The listing builds one solid part. Answer for the finished solid, in the listing's coordinates (mm). A direction names the side the tool comes from. Round coordinates to 2 decimals unless told otherwise and drop trailing zeros. Order: outer loops, then holes, each group sorted by start corner. A loop starts at its lowest first (then second) coordinate and runs counter-clockwise, first axis right, second up. Notation, with made-up numbers: (-17, 18.5) -> (19, 18.5) arc R30 cw to (19, 47.5) -> close; hole circle Ø4 at (47, 45.25). An arc over 180 degrees is marked (long way). Return JSON: item names as keys, results as strings. Group by question number.
(1) The part is cut by section D-D (z = 20.01). Determine the outline of the cut face in (x, y).
(2) Which of the six approach directions +Z, -Z, +X, -X, +Y, -Y give full straight-line access (tool end or side, diameter ignored) to faces 1 (the face through (0, 17, 17)), 2 (the face through (0, 3, -20)), 3 (the face through (0, 1, 17)), 4 (the face through (0.1, 5.9, 7.5)), 5 (the face through (0, 4.5, -20))?
(3) Each of these flat-tipped pins is pushed along its axis until it touches: pin 1 (2.5 mm diameter, centred on x = 3, z = 19, fed in from +Y); pin 2 (2.5 mm diameter, centred on x = -2, y = 1.5, fed in from -Z); pin 3 (1.8 mm diameter, centred on x = -4.55, z = 20.01, fed in from -Y); pin 4 (1 mm diameter, centred on x = -0.5, y = 27, fed in from +Z). Where does it stop, or does it pass through?
(4) The part is cut by section B-B (z = 10). Determine the outline of the cut face in (x, y), plus the area to 3 significant figures.
(5) The part is cut by section C-C (x = 0). Determine the outline of the cut face in (y, z).
(6) Consider line 1 (X direction, y = 3.7, z = 20.01); line 2 (Z direction, x = -0.75, y = 14.5); line 3 (X direction, y = 4.5, z = 10). Determine where each line is inside the solid, lowest interval first. Write a range as [from, to].
(7) Determine the mould class of faces 6 (the face through (6.724, 3.74, 19.527)), 7 (the face through (0, 4, 22)), 8 (the face through (5.56, 3.74, -21.12)) for opening direction X: +X half, -X half, draft (parallel to the pull), parting line (faces both ways), or undercut.
(8) The part is cut by section A-A (x = 4.55). Determine the outline of the cut face in (y, z).
from build123d import *

# Parameters (mm, degrees)
SKETCH1_W           = 14
SKETCH1_H           = 34
SKETCH1_R           = 2.5
BOSS_EXTRUDE1_DEPTH = 30
SKETCH1_3_R         = 2.5
CUT_EXTRUDE1_DEPTH  = 12
BOSS_EXTRUDE2_START = -3
SKETCH4_R           = 1.5
BOSS_EXTRUDE2_DEPTH = 1.5


with BuildPart() as part:
    # Sketch1 → Boss-Extrude1 (new body)
    with BuildSketch(Plane(origin=(0, 0, 0), x_dir=(1, 0, 0), z_dir=(0, 1, 0))):
        Rectangle(SKETCH1_W, SKETCH1_H)
        with Locations((0, -10)):
            Circle(SKETCH1_R, mode=Mode.SUBTRACT)
        with Locations((0, -10)):
            Circle(SKETCH1_R)
    extrude(amount=BOSS_EXTRUDE1_DEPTH)

    # Sketch1_3 → Cut-Extrude1 (cut)
    with BuildSketch(Plane(origin=(0, 0, 0), x_dir=(1, 0, 0), z_dir=(0, 1, 0))):
        with Locations(Location((0, -10, 0), (0, 0, 270))):
            Circle(SKETCH1_3_R)
    extrude(amount=CUT_EXTRUDE1_DEPTH, mode=Mode.SUBTRACT)

    # Sketch4 → Boss-Extrude2 (add)
    with BuildSketch(Plane.XZ.offset(BOSS_EXTRUDE2_START)):
        with BuildLine():
            Line((0, 22), (-5.877806956, 22))
            ThreePointArc((-5.877806956, 22), (-6.716005023, 19.562192285), (-7, 17))
            Line((-7, 17), (0, 17))
            Line((0, 17), (0, 22))
        make_face()
        with Locations(Location((-4.55, 20.01, 0), (0, 0, 270))):
            Circle(SKETCH4_R, mode=Mode.SUBTRACT)
        with BuildLine():
            Line((5.877806956, 22), (0, 22))
            Line((0, 22), (0, 17))
            Line((0, 17), (7, 17))
            ThreePointArc((7, 17), (6.716005023, 19.562192285), (5.877806956, 22))
        make_face()
        with Locations(Location((4.55, 20.01, 0), (0, 0, 270))):
            Circle(SKETCH4_R, mode=Mode.SUBTRACT)
    boss_extrude2 = extrude(amount=-BOSS_EXTRUDE2_DEPTH)

    # Mirror1: Boss-Extrude2 across plane
    add(boss_extrude2.mirror(Plane.XY))


solid = part.part
Answer below:
{
 "1": {"outline": "(-6.61, 3) -> (-6.05, 3) -> (-6.05, 4.5) -> (-6.61, 4.5) -> close; (-3.05, 3) -> (3.05, 3) -> (3.05, 4.5) -> (-3.05, 4.5) -> close; (6.05, 3) -> (6.61, 3) -> (6.61, 4.5) -> (6.05, 4.5) -> close"},
 "2": {"face 1": "+Z, +X, -X, +Y", "face 2": "-Z, +X, -X, -Y", "face 3": "+Z, +X, -X, -Y", "face 4": "-Y", "face 5": "-Z, +X, -X, +Y"},
 "3": {"pin 1": "stops at y = 4.5", "pin 2": "stops at z = -17", "pin 3": "passes through", "pin 4": "stops at z = 17"},
 "4": {"outline": "(-7, 0) -> (-2.5, 0) -> (-2.5, 12) -> (2.5, 12) -> (2.5, 0) -> (7, 0) -> (7, 30) -> (-7, 30) -> close", "area": "360 mm²"},
 "5": {"outline": "(0, -17) -> (3, -17) -> (3, -22) -> (4.5, -22) -> (4.5, -17) -> (30, -17) -> (30, 17) -> (4.5, 17) -> (4.5, 22) -> (3, 22) -> (3, 17) -> (0, 17) -> (0, 12.5) -> (12, 12.5) -> (12, 7.5) -> (0, 7.5) -> close"},
 "6": {"line 1": "x = [-6.61, -6.05], [-3.05, 3.05], [6.05, 6.61]", "line 2": "z = [-17, 17]", "line 3": "x = [-7, -2.5], [2.5, 7]"},
 "7": {"face 6": "+X half", "face 7": "draft", "face 8": "undercut"},
 "8": {"outline": "(0, -17) -> (3, -17) -> (3, -18.51) -> (4.5, -18.51) -> (4.5, -17) -> (30, -17) -> (30, 17) -> (4.5, 17) -> (4.5, 18.51) -> (3, 18.51) -> (3, 17) -> (0, 17) -> close; (3, -22) -> (4.5, -22) -> (4.5, -21.51) -> (3, -21.51) -> close; (3, 21.51) -> (4.5, 21.51) -> (4.5, 22) -> (3, 22) -> close"}
}
